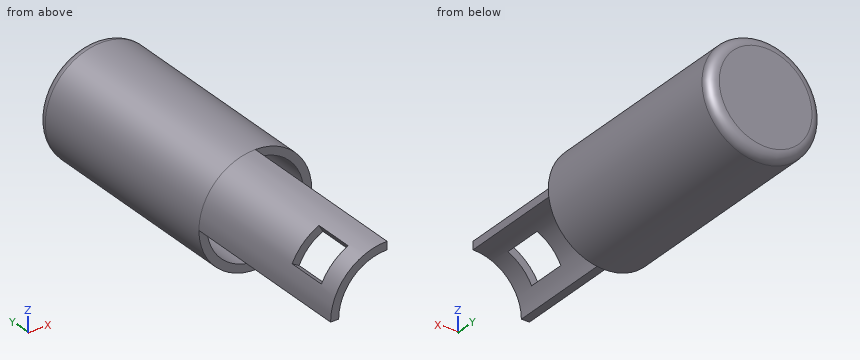
from build123d import *

# Parameters (mm, degrees)
F0_R      = 14
F1_DEPTH  = 55
F2_R      = 12
F3_DEPTH  = 25
F4_R      = 11
F5_DEPTH  = 20
F6_R      = 2.5
F10_DEPTH = 45
F12_START = -5
F12_DEPTH = 10


with BuildPart() as f1:
    # F0 (on Front) → F1 (new body)
    with BuildSketch(Plane.XZ):
        Circle(F0_R)
    extrude(amount=F1_DEPTH)

    # F2 (on face) → F3 (cut)
    with BuildSketch(Plane.XZ.offset(55)):
        Circle(F2_R)
    extrude(amount=-F3_DEPTH, mode=Mode.SUBTRACT)

    # F4 (on face) → F5 (cut)
    with BuildSketch(Plane.XZ.offset(30)):
        Circle(F4_R)
    extrude(amount=-F5_DEPTH, mode=Mode.SUBTRACT)

    # F6
    f6_edges = [f1.edges().sort_by_distance(p)[0] for p in [
        (-14, 0, 0),
    ]]
    fillet(f6_edges, radius=F6_R)

    # F7 (on Top) → F8 (revolve)
    with BuildSketch(Plane.XY):
        Polygon((0, -21), (0, -10), (-11, -10), align=None)
    revolve(axis=Axis((0, -15.5, 0), (0, -1, 0)))

    # F9 (on face) → F10 (join)
    with BuildSketch(Plane.XZ.offset(55)):
        with BuildLine():
            Line((-14, 0), (-12, 0))
            ThreePointArc((-12, 0), (-8.4852813742, 8.4852813742), (0, 12))
            Line((0, 12), (0, 14))
            ThreePointArc((0, 14), (-9.8994949366, 9.8994949366), (-14, 0))
        make_face()
    extrude(amount=F10_DEPTH)

    # F11 (on face) → F12 (cut)
    with BuildSketch(Plane.XZ.offset(100).offset(F12_START)):
        with BuildLine():
            Line((-12.6491106407, 6), (-10.9087121146, 5))
            ThreePointArc((-10.9087121146, 5), (-8.4852813742, 8.4852813742), (-5, 10.9087121146))
            Line((-5, 10.9087121146), (-6, 12.6491106407))
            ThreePointArc((-6, 12.6491106407), (-9.8994949366, 9.8994949366), (-12.6491106407, 6))
        make_face()
    extrude(amount=-F12_DEPTH, mode=Mode.SUBTRACT)


solid = f1.part
Geometry: final body of the model. Coordinates: model frame, mm. Coordinates: 2 decimals unless noted, no trailing zeros. Write each loop counter-clockwise with the first axis right and the second up, starting at its lowest first coordinate (ties: lowest second). Pieces come first, ordered by that corner, then holes. Notation, with made-up numbers: (14, 50.25) - (37, 50.25) arc R15 cw to (37, 75.25) - close; hole circle Ø9 at (-7, 45). An arc over 180 degrees is marked (long way). Return JSON: item names as keys, results as strings.
Item 1: Section query B-B (y = -53). Output: boundary loops of the cut face in (x, z).
Completed:
{"outline": "circle Ø28 at (0, 0); hole circle Ø24 at (0, 0)"}
Item 2: Section query A-A (y = -93). Output: boundary loops of the cut face in (x, z).
Completed:
{"outline": "(-14, 0) - (-12, 0) arc R12 cw to (-10.91, 5) - (-12.65, 6) arc R14 ccw to start; (-6, 12.65) - (-5, 10.91) arc R12 cw to (0, 12) - (0, 14) arc R14 ccw to start"}
Item 3: Line query: L1, parallel to Z at x = 0, y = -48.75; L2, parallel to X at y = -23.25, z = 0. Output: solid intervals per line, ascending.
Completed:
{"L1": "z = -14 to -12, 12 to 14", "L2": "x = -14 to -11, 11 to 14"}
Item 4: Pin query (flat end, axial travel): pin 1 Ø1 at (x, y) = (-12.5, -70.5) entering from -Z; pin 2 Ø5 at (y, z) = (-55, 4.5) entering from +X; pin 3 Ø1.5 at (y, z) = (-51, -7.5) entering from +X; pin 4 Ø4 at (y, z) = (-87.5, 8.5) entering from +X (3 decimals). Return the tip coordinate at first contact, or that it passes through.
Completed:
{"pin 1": "stops at z = 0", "pin 2": "stops at x = 13.86", "pin 3": "stops at x = 12.27", "pin 4": "passes through"}
